Autodesk Inventor part; units mm, degrees
ref_plane "YZ Plane" through (0, 0, 0) normal (1, 0, 0) x (0, 1, 0)
ref_plane "XZ Plane" through (0, 0, 0) normal (0, 1, 0) x (-1, 0, 0)
ref_plane "XY Plane" through (0, 0, 0) normal (0, 0, 1) x (1, 0, 0)
sketch "Sketch1" plane through (0, 0, 0) normal (0, 0, 1) x (1, 0, 0)
  point P0 (0, 0)
sketch "Sketch2" plane through (0, 0, 0) normal (0, 0, 1) x (1, 0, 0)
  line L0 (22, -17) -> (-22, -17)
  line L1 (-22, -17) -> (-22, 17)
  line L2 (-22, 17) -> (22, 17)
  line L3 (22, 17) -> (22, -17)
  line L4 (22, -17) -> (-22, 17) construction
  line L5 (-22, -17) -> (22, 17) construction
  line L6 (25.0001, -20) -> (-25.0001, -20)
  line L7 (-25.0001, -20) -> (-25.0001, 20)
  line L8 (-25.0001, 20) -> (25.0001, 20)
  line L9 (25.0001, 20) -> (25.0001, -20)
  line L10 (25.0001, -20) -> (-25.0001, 20) construction
  line L11 (-25.0001, -20) -> (25.0001, 20) construction
  point P0 (0, 0)
extrude "Extrusion1" add sketch "Sketch2" along normal blind 80
properties part number "enclosure_80x40x50_mm"
Input: part model. Units: mm. Frame: model coordinates. A direction names the side the tool comes from. Coordinates: 2 decimals unless noted, no trailing zeros. Loops run counter-clockwise (first coordinate to the right, second up) from the corner with the lowest first, then second, coordinate; pieces in that order, holes last. Notation, with made-up numbers: (-8.5, -24) - (14.5, -24) arc R4 cw to (14.5, -20) - close; hole circle Ø6 at (51, 75). An arc over 180 degrees is marked (long way). Answer in a Markdown table with one row per item.
(1) Cut plane C-C on y = -11. Output: boundary loops of the cut face in (x, z), plus the area to 3 significant figures.
Model answer:
| item | result |
|---|---|
| outline | (-25, 0) - (-22, 0) - (-22, 80) - (-25, 80) - close; (22, 0) - (25, 0) - (25, 80) - (22, 80) - close |
| area | 480 mm² |
(2) Cut plane B-B on z = 16.5. Output: boundary loops of the cut face in (x, y), plus the area to 3 significant figures.
Model answer:
| item | result |
|---|---|
| outline | (-25, -20) - (25, -20) - (25, 20) - (-25, 20) - close; hole (-22, -17) - (22, -17) - (22, 17) - (-22, 17) - close |
| area | 504 mm² |
(3) Cut plane A-A on x = 17. Output: boundary loops of the cut face in (y, z).
Model answer:
| item | result |
|---|---|
| outline | (-20, 0) - (-17, 0) - (-17, 80) - (-20, 80) - close; (17, 0) - (20, 0) - (20, 80) - (17, 80) - close |
(4) Mould query, pull axis Y, two halves, no side actions, for faces 3 (the face through (0, -17, 39)), 4 (the face through (0, 20, 39)), 5 (the face through (0, 18, 0)). Classes: pulls with the +Y half, pulls with the -Y half, needs draft (parallel to the pull), parting line crosses it, or undercut.
Model answer:
| item | result |
|---|---|
| face 3 | undercut |
| face 4 | pulls with the +Y half |
| face 5 | needs draft |
(5) Material intervals for L1, parallel to Y at x = -17, z = 59.5; L2, parallel to X at y = 2.5, z = 40.5, sorted ascending. Write a range as from..to.
Model answer:
| item | result |
|---|---|
| L1 | y = -20..-17, 17..20 |
| L2 | x = -25..-22, 22..25 |
(6) Set-up query: faces 1 (the face through (0, -20, 39)), 2 (the face through (-22, 0, 39)). Return all of +Z, -Z, +X, -X, +Y, -Y with unobstructed straight access to the full face (end or side cutting, diameter ignored); none if empty.
Model answer:
| item | result |
|---|---|
| face 1 | +Z, -Z, +X, -X, -Y |
| face 2 | +Z, -Z |
